Could you check a few things on this model? Use its own coordinates, in mm. Face numbers are marked on the shaded views. A direction names the side the tool comes from. Give positions to 0.01 mm unless a question says otherwise; leave off trailing zeros. Loops run counter-clockwise (first coordinate to the right, second up) from the corner with the lowest first, then second, coordinate; pieces in that order, holes last.
1. Imagine slicing it at D-D (y = 54). List the corners of the cut face in (x, z) for me, plus the area to 3 significant figures.
2. Thinking about a two-plate mould opening in Y: for the marked faces 1, 2 and 3, which applies, +Y half, -Y half, draft (parallel to the pull), parting line (faces both ways), or undercut?
3. Imagine slicing it at A-A (y = 0). List the corners of the cut face in (x, z) for me, plus the area to 3 significant figures.
4. Imagine slicing it at C-C (z = -0.9). List the corners of the cut face in (x, y) for me.
5. I need wall thicknesses on line 1 along Y through (x, z) = (0, 1.1); line 2 along X through (y, z) = (49.5, -0.7); line 3 along X through (y, z) = (-7, 1.05). Which ranges of each line are inside material? Lowest first, please.
6. For P1, Ø3, axis at y = 16, z = 0, coming from the -X side; P2, Ø2, axis at x = -7.5, z = -1.5, coming from the +Y side; P3, Ø1, axis at y = -4, z = 0.5, coming from the -X side, each with a flat end and sliding along its axis, tell me the tip position at first contact or that it passes through.
7. Imagine slicing it at B-B (x = 0). List the corners of the cut face in (y, z) for me.
8. For the marked faces 4, 5 and 6, which set-ups out of +Z, -Z, +X, -X, +Y, -Y let a thin tool reach every point of the face, with its end or its side?
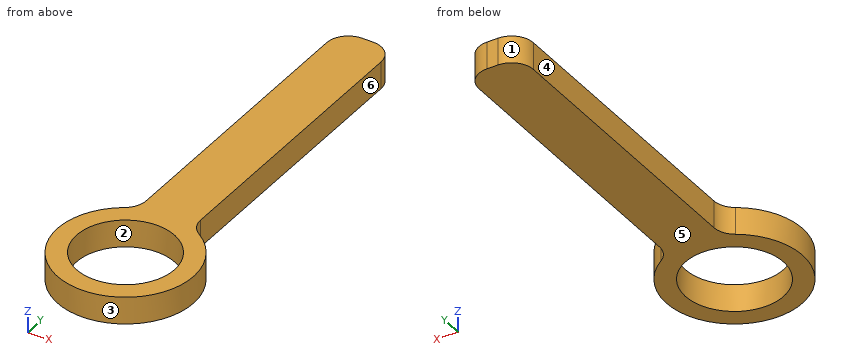
```python
from build123d import *

# Parameters (mm, degrees)
SKETCH1_R           = 9
BOSS_EXTRUDE1_DEPTH = 2.5


with BuildPart() as part:
    # Sketch1 → Boss-Extrude1 (new, symmetric)
    with BuildSketch(Plane.XY):
        with BuildLine():
            Line((-5, 13.829316686), (-5, 66))
            ThreePointArc((-5, 66), (-3.828427125, 68.828427125), (-1, 70))
            Line((-1, 70), (1, 70))
            ThreePointArc((1, 70), (3.828427125, 68.828427125), (5, 66))
            Line((5, 66), (5, 13.829316686))
            ThreePointArc((5, 13.829316686), (5.483803708, 11.922391507), (6.818181818, 10.476755065))
            ThreePointArc((6.818181818, 10.476755065), (0, -12.5), (-6.818181818, 10.476755065))
            ThreePointArc((-6.818181818, 10.476755065), (-5.483803708, 11.922391507), (-5, 13.829316686))
        make_face()
        Circle(SKETCH1_R, mode=Mode.SUBTRACT)
    extrude(amount=BOSS_EXTRUDE1_DEPTH, both=True)


solid = part.part
```
Derived:
1. outline: (-5, -2.5) - (5, -2.5) - (5, 2.5) - (-5, 2.5) - close
1. area: 50.0 mm2
2. face 1: +Y half
2. face 2: undercut
2. face 3: parting line
3. outline: (-12.5, -2.5) - (-9, -2.5) - (-9, 2.5) - (-12.5, 2.5) - close; (9, -2.5) - (12.5, -2.5) - (12.5, 2.5) - (9, 2.5) - close
3. area: 35.0 mm2
4. outline: (-6.82, 10.48) arc R12.5 ccw (long way) to (6.82, 10.48) arc R4 cw to (5, 13.83) - (5, 66) arc R4 ccw to (1, 70) - (-1, 70) arc R4 ccw to (-5, 66) - (-5, 13.83) arc R4 cw to start; hole circle Ø18 at (0, 0)
5. line 1: y = -12.5 to -9, 9 to 70
5. line 2: x = -5 to 5
5. line 3: x = -10.36 to -5.66, 5.66 to 10.36
6. P1: stops at x = -5
6. P2: stops at y = 10.71
6. P3: stops at x = -12
7. outline: (-12.5, -2.5) - (-9, -2.5) - (-9, 2.5) - (-12.5, 2.5) - close; (9, -2.5) - (70, -2.5) - (70, 2.5) - (9, 2.5) - close
8. face 4: +Z, -Z, -X, +Y
8. face 5: -Z, +X, -X, +Y, -Y
8. face 6: +Z, -Z, +X, +Y
